Geometry check sheet. Reference: the model listing, model coordinates, mm. Face numbers are marked on the shaded views. A direction names the side the tool comes from. Coordinates: 2 decimals unless noted, no trailing zeros. Write each loop counter-clockwise with the first axis right and the second up, starting at its lowest first coordinate (ties: lowest second). Pieces come first, ordered by that corner, then holes. Notation, with made-up numbers: (30.25, 37) -> (65.25, 37) arc R36 cw to (65.25, 71) -> close; hole circle Ø2 at (34, 6). An arc over 180 degrees is marked (long way). One line per question, with ' | ' between items.
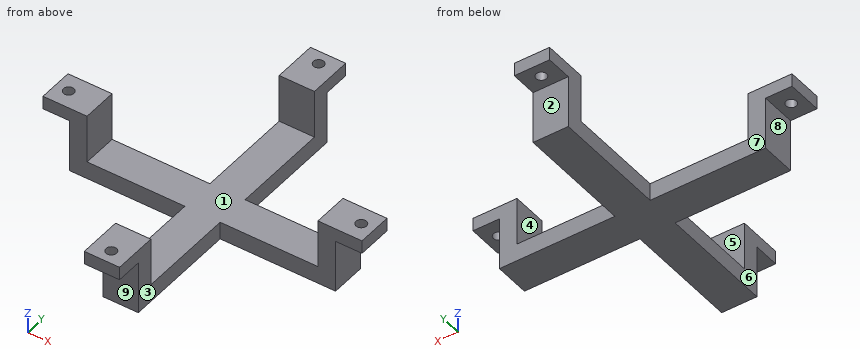
```python
from build123d import *

# Parameters (mm, degrees)
SKETCH_1_W      = 26.2
SKETCH_1_H      = 4
SKETCH_1_W_2    = 4
SKETCH_1_H_2    = 26.2
EXTRUDE_1_DEPTH = 2
SKETCH_1_6_W    = 2
SKETCH_1_6_H    = 4
SKETCH_1_6_W_2  = 4
SKETCH_1_6_H_2  = 2
EXTRUDE_2_DEPTH = 7.5
EXTRUDE_START   = 7.5
SKETCH_1_7_W    = 3
SKETCH_1_7_H    = 4
SKETCH_1_7_R    = 0.6
SKETCH_1_7_W_2  = 4
SKETCH_1_7_H_2  = 3
EXTRUDE_3_DEPTH = 1.5


with BuildPart() as part:
    # 草图1 → 凸台-拉伸1 (new body)
    with BuildSketch(Plane.XY):
        Rectangle(SKETCH_1_W, SKETCH_1_H)
        Rectangle(SKETCH_1_W_2, SKETCH_1_H_2)
    extrude(amount=EXTRUDE_1_DEPTH)

    # 草图1<6> → 凸台-拉伸2 (add)
    with BuildSketch(Plane.XY):
        with Locations((14.1, 0)):
            Rectangle(SKETCH_1_6_W, SKETCH_1_6_H)
        with Locations((0, 14.1)):
            Rectangle(SKETCH_1_6_W_2, SKETCH_1_6_H_2)
        with Locations((0, -14.1)):
            Rectangle(SKETCH_1_6_W_2, SKETCH_1_6_H_2)
        with Locations((-14.1, 0)):
            Rectangle(SKETCH_1_6_W, SKETCH_1_6_H)
    extrude(amount=EXTRUDE_2_DEPTH)

    # 草图1<7> → 凸台-拉伸3 (add)
    # profile 1 of 4: a face of its own
    with BuildSketch(Plane.XY.offset(EXTRUDE_START)):
        with Locations((-16.6, 0)):
            Rectangle(SKETCH_1_7_W, SKETCH_1_7_H)
        with Locations((-16.6, 0)):
            Circle(SKETCH_1_7_R, mode=Mode.SUBTRACT)
    # profile 2 of 4: a face of its own
    with BuildSketch(Plane.XY.offset(EXTRUDE_START)):
        with Locations((0, 16.6)):
            Rectangle(SKETCH_1_7_W_2, SKETCH_1_7_H_2)
        with Locations((0, 16.6)):
            Circle(SKETCH_1_7_R, mode=Mode.SUBTRACT)
    # profile 3 of 4: a face of its own
    with BuildSketch(Plane.XY.offset(EXTRUDE_START)):
        with Locations((16.6, 0)):
            Rectangle(SKETCH_1_7_W, SKETCH_1_7_H)
        with Locations((16.6, 0)):
            Circle(SKETCH_1_7_R, mode=Mode.SUBTRACT)
    # profile 4 of 4: a face of its own
    with BuildSketch(Plane.XY.offset(EXTRUDE_START)):
        with Locations((0, -16.6)):
            Rectangle(SKETCH_1_7_W_2, SKETCH_1_7_H_2)
        with Locations((0, -16.6)):
            Circle(SKETCH_1_7_R, mode=Mode.SUBTRACT)
    extrude(amount=-EXTRUDE_3_DEPTH)


solid = part.part
```
(1) Cross-section at A-A (y = 16.6). Record the cut outline in (x, z), plus the area to 3 significant figures.
Answers below:
outline: (-2, 6) -> (-0.6, 6) -> (-0.6, 7.5) -> (-2, 7.5) -> close; (0.6, 6) -> (2, 6) -> (2, 7.5) -> (0.6, 7.5) -> close | area: 4.20 mm²
(2) Cross-section at D-D (y = 0). Record the cut outline in (x, z).
Answers below:
outline: (-18.1, 6) -> (-17.2, 6) -> (-17.2, 7.5) -> (-18.1, 7.5) -> close; (-16, 6) -> (-15.1, 6) -> (-15.1, 0) -> (15.1, 0) -> (15.1, 6) -> (16, 6) -> (16, 7.5) -> (13.1, 7.5) -> (13.1, 2) -> (-13.1, 2) -> (-13.1, 7.5) -> (-16, 7.5) -> close; (17.2, 6) -> (18.1, 6) -> (18.1, 7.5) -> (17.2, 7.5) -> close
(3) Depth check by flat-ended pin: P1, Ø1, axis at x = 0, z = 1, coming from the +Y side; P2, Ø1.2, axis at y = 0.5, z = 1.5, coming from the -X side; P3, Ø4, axis at x = 10, z = 2.5, coming from the +Y side; P4, Ø2, axis at x = -8, z = 3.5, coming from the -Y side. Enter the tip coordinate at first touch or a pass-through.
Answers below:
P1: stops at y = 15.1 | P2: stops at x = -15.1 | P3: stops at y = 2 | P4: passes through
(4) Cross-section at C-C (z = 2.75). Record the cut outline in (x, y), plus the area to 3 significant figures.
Answers below:
outline: (-15.1, -2) -> (-13.1, -2) -> (-13.1, 2) -> (-15.1, 2) -> close; (-2, -15.1) -> (2, -15.1) -> (2, -13.1) -> (-2, -13.1) -> close; (-2, 13.1) -> (2, 13.1) -> (2, 15.1) -> (-2, 15.1) -> close; (13.1, -2) -> (15.1, -2) -> (15.1, 2) -> (13.1, 2) -> close | area: 32.0 mm²
(5) Material ranges on line 1 (Y direction, x = -16.6, z = 6.85); line 2 (Y direction, x = -7, z = 1.25), recorded low to high.
Answers below:
line 1: y = -2 to -0.6, 0.6 to 2 | line 2: y = -2 to 2
(6) Tool access check on the marked faces 5, 6, 7, 8 and 9. Record the directions out of +Z, -Z, +X, -X, +Y, -Y that give a thin tool (end or side, any length) a straight path to the whole face; none if there is none.
Answers below:
face 5: +Z, +X, -X | face 6: +Z, -Z, -X, -Y | face 7: +Z, -Z, -X, +Y | face 8: -Z, -X, +Y, -Y | face 9: -Z, +X, -X, -Y
(7) Draft check along X on the marked faces 1, 2, 3 and 4. Enter one of: pulls with the +X half, pulls with the -X half, needs draft (parallel to the pull), parting line crosses it, or undercut.
Answers below:
face 1: undercut | face 2: needs draft | face 3: pulls with the +X half | face 4: undercut
